Input: part model. Units: mm. Frame: model coordinates. A direction names the side the tool comes from. Give positions to 0.01 mm unless a question says otherwise; leave off trailing zeros. Loops run counter-clockwise (first coordinate to the right, second up) from the corner with the lowest first, then second, coordinate; pieces in that order, holes last. Notation, with made-up numbers: (28.5, 77.25) - (53.5, 77.25) arc R18 ccw to (53.5, 92.25) - close; hole circle Ø6 at (59, 20). An arc over 180 degrees is marked (long way). Answer as a JSON object with one key per item and string values. Group by question number.
(1) Material intervals for L1, parallel to Y at x = 11, z = -17.5; L2, parallel to X at y = -9, z = -23; L3, parallel to Y at x = 25, z = -11.5, sorted ascending.
(2) Mould query, pull axis Z, two halves, no side actions, for faces 1 (the cylindrical face through (-0.69, -66.08, -3.1)), 2 (the flat face through (1.4, -120.65, -2.1)), 3 (the flat face through (10, -3.81, -10)). Classes: +Z half, -Z half, draft (parallel to the pull), parting line (faces both ways), or undercut.
(3) Section query A-A (x = 0). Return loops of the section in (y, z) (3 decimals), plus the area to 3 significant figures.
(4) Section query C-C (y = -62). Return loops of the section in (x, z) (3 decimals).
(5) Pin query (flat end, axial travel): P1, Ø5, axis at y = -65, z = -2.5, coming from the +X side (3 decimals); P2, Ø1, axis at x = -1, z = -16, coming from the -Y side. Return the tip coordinate at first contact, or that it passes through.
(6) Access query for faces 4 (the flat face through (0, -124.46, 0)), 5 (the cylindrical face through (-0.5, -122.58, -2.23)). Directions: +Z, -Z, +X, -X, +Y, -Y. A direction counts if a zero-diameter tool reaches every point of the face in a straight line with its end or side. Return the directions, or none.
(7) Section query B-B (z = 0). Return loops of the section in (x, y) (3 decimals).
```python
from build123d import *

# Parameters (mm, degrees)
F0_R     = 31.75
F0_R_2   = 3.175
F1_DEPTH = 3.81
F2_DEPTH = 124.46
F0_R_3   = 34.925
F3_DEPTH = 12.7
F5_R     = 3.175
F5_R_2   = 2.286
F6_DEPTH = 3.81


# Not quite as in the source:
# - a fillet or chamfer that OpenCascade refuses, or shapes differently, is made with other operations: its cross-section is extruded or revolved along the edge and cut away or added


with BuildPart() as f1:
    # F0 (on Front) → F1 (new body)
    with BuildSketch(Plane.XZ):
        Circle(F0_R)
        Circle(F0_R_2, mode=Mode.SUBTRACT)
        Circle(F0_R_2)
    extrude(amount=F1_DEPTH)

    # F0 (on Front) → F2 (join)
    with BuildSketch(Plane.XZ):
        Circle(F0_R_2)
    extrude(amount=F2_DEPTH)

    # F0 (on Front) → F3 (join)
    with BuildSketch(Plane.XZ):
        Circle(F0_R_3)
        Circle(F0_R, mode=Mode.SUBTRACT)
    extrude(amount=F3_DEPTH)

    # F4: fillet of radius 9.1981536726 on 3 edges, made by hand

    # F4_s1 → F4_t2 (revolve)
    with BuildSketch(Plane.XY):
        with BuildLine():
            ThreePointArc((31.75, -12.7), (28.9512095664, -6.3960255802), (22.5570096106, -3.81))
            Line((22.5570096106, -3.81), (31.75, -3.81))
            Line((31.75, -3.81), (31.75, -12.7))
        make_face()
    revolve(axis=Axis((0, -3.81, 0), (0, -1, 0)))

    # F4_s3 → F4_t4 (revolve)
    with BuildSketch(Plane.XY):
        with BuildLine():
            ThreePointArc((12.3731536726, -3.81), (5.8690768363, -6.5040768363), (3.175, -13.0081536726))
            Line((3.175, -13.0081536726), (3.175, -3.81))
            Line((3.175, -3.81), (12.3731536726, -3.81))
        make_face()
    revolve(axis=Axis((0, -3.81, 0), (0, 1, 0)))

    # F4_s5 → F4_t6 (revolve, cut)
    with BuildSketch(Plane.XY):
        with BuildLine():
            ThreePointArc((34.925, -5.7481908239), (34.0936833659, -9.5694561844), (31.75, -12.7))
            Line((31.75, -12.7), (34.925, -12.7))
            Line((34.925, -12.7), (34.925, -5.7481908239))
        make_face()
    revolve(axis=Axis((0, -12.7, 0), (0, -1, 0)), mode=Mode.SUBTRACT)

    # F5 (on face) → F6 (cut)
    with BuildSketch(Plane.XZ.offset(124.46)):
        Circle(F5_R)
        Circle(F5_R_2, mode=Mode.SUBTRACT)
    extrude(amount=-F6_DEPTH, mode=Mode.SUBTRACT)


solid = f1.part
```
Recorded:
{
 "1": {"L1": "y = -3.81 to 0", "L2": "x = -25.49 to -20.54, 20.54 to 25.49", "L3": "y = -5.26 to 0"},
 "2": {"face 1": "parting line", "face 2": "draft", "face 3": "undercut"},
 "3": {"outline": "(-124.46, -2.286) - (-120.65, -2.286) - (-120.65, -3.175) - (-13.008, -3.175) arc R9.198 cw to (-3.81, -12.373) - (-3.81, -22.557) arc R9.198 cw to (-12.7, -31.75) arc R9.198 ccw to (-5.748, -34.925) - (0, -34.925) - (0, 34.925) - (-5.748, 34.925) arc R9.198 ccw to (-12.7, 31.75) arc R9.198 cw to (-3.81, 22.557) - (-3.81, 12.373) arc R9.198 cw to (-13.008, 3.175) - (-120.65, 3.175) - (-120.65, 2.286) - (-124.46, 2.286) - close", "area": "1,140 mm^2"},
 "4": {"outline": "circle Ø6.35 at (0, 0)"},
 "5": {"P1": "stops at x = 3.175", "P2": "stops at y = -3.81"},
 "6": {"face 4": "+Z, -Z, +X, -X, -Y", "face 5": "-Y"},
 "7": {"outline": "(-34.925, -5.748) arc R9.198 ccw to (-31.75, -12.7) arc R9.198 cw to (-22.557, -3.81) - (-12.373, -3.81) arc R9.198 cw to (-3.175, -13.008) - (-3.175, -120.65) - (-2.286, -120.65) - (-2.286, -124.46) - (2.286, -124.46) - (2.286, -120.65) - (3.175, -120.65) - (3.175, -13.008) arc R9.198 cw to (12.373, -3.81) - (22.557, -3.81) arc R9.198 cw to (31.75, -12.7) arc R9.198 ccw to (34.925, -5.748) - (34.925, 0) - (-34.925, 0) - close"}
}
